```python
from build123d import *

# Parameters (mm, degrees)
F0_R     = 5
F1_DEPTH = 33
F2_R     = 4.9
F3_DEPTH = 16
F4_SIZE2 = 15.99999
F4_SIZE  = 4.49999
F5_R     = 6
F5_R_2   = 5
F6_DEPTH = 83
F7_R     = 5


# Not quite as in the source:
# - a fillet or chamfer is up to 0.001 mm smaller than in the source, because OpenCascade refuses the exact size


with BuildPart() as f1:
    # F0 (on Top) → F1 (new body)
    with BuildSketch(Plane.XY):
        Circle(F0_R)
    extrude(amount=F1_DEPTH)

    # F2 (on face) → F3 (join)
    with BuildSketch(Plane(origin=(0, 0, 0), x_dir=(1, 0, 0), z_dir=(0, 0, -1))):
        Circle(F2_R)
    extrude(amount=F3_DEPTH)

    # F4 (size 4.5 and 16 in the source; OpenCascade refuses exactly that, so slightly less here)
    f4_edges = [f1.edges().sort_by_distance(p)[0] for p in [
        (-4.9, 0, -16),
    ]]
    f4_side = f1.faces().sort_by_distance((0, 0, -16))[0]
    chamfer(f4_edges, length=F4_SIZE, length2=F4_SIZE2, reference=f4_side)

    # F5 (on face) → F6 (join)
    with BuildSketch(Plane.XY.offset(33)):
        Circle(F5_R)
        Circle(F5_R_2, mode=Mode.SUBTRACT)
        Circle(F5_R_2)
    extrude(amount=F6_DEPTH)

    # F7
    f7_edges = [f1.edges().sort_by_distance(p)[0] for p in [
        (-6, 0, 116),
    ]]
    fillet(f7_edges, radius=F7_R)


solid = f1.part
```
The listing builds one solid part. Answer for the finished solid, in the listing's coordinates (mm). A direction names the side the tool comes from. Round coordinates to 2 decimals unless told otherwise and drop trailing zeros. Write each loop counter-clockwise with the first axis right and the second up, starting at its lowest first coordinate (ties: lowest second). Pieces come first, ordered by that corner, then holes. Notation, with made-up numbers: (23, 9.25) -> (57, 9.25) arc R23 ccw to (57, 29.25) -> close; hole circle Ø10 at (54.25, 33). An arc over 180 degrees is marked (long way). Write item = value, one per line.
1) For a pull along X with two mould halves and no side action, classify faces 3 (the conical face through (-0.581, 2.618, -7.888)), 4 (the flat face through (0, 0, 116)) as released by +X, released by -X, zero draft, split by the parting line, or undercut.
Check values:
face_3 = split by the parting line
face_4 = zero draft
2) Given pin 1 (1.5 mm diameter, centred on x = -3, z = 10, fed in from +Y); pin 2 (6 mm diameter, centred on y = 4.5, z = 86.5, fed in from +X); pin 3 (6 mm diameter, centred on x = 1, z = 17, fed in from +Y), each flat-ended and moving along its own axis, determine where each tip first touches the part or whether it passes through.
Check values:
pin_1 = 4.47
pin_2 = 5.81
pin_3 = 5
3) Section A-A on z = 51.5 is taken. Write down the section's boundary in (x, y).
Check values:
outline = circle Ø12 at (0, 0)
4) Section B-B on z = 11.5 is taken. Write down the section's boundary in (x, y), plus the area to 3 significant figures.
Check values:
outline = circle Ø10 at (0, 0)
area = 78.5 mm²
5) Straight lines are drawn through the part: line 1 along Y through (x, z) = (3.5, 74); line 2 along Y through (x, z) = (-0.5, 96.5); line 3 along Z through (x, y) = (-4.5, -3). For each, find the intervals that lie inside material, in ascending order. Write a range as [from, to].
Check values:
line_1 = [-4.87, 4.87]
line_2 = [-5.98, 5.98]
line_3 = [33, 113.36]
6) Which of the six approach directions +Z, -Z, +X, -X, +Y, -Y give full straight-line access (tool end or side, diameter ignored) to faces 1 (the cylindrical face through (-6, 0, 71)), 2 (the cylindrical face through (-1.08, -4.88, 16.27))?
Check values:
face_1 = +Z, -Z
face_2 = -Z
